Drawing for the job (mm, zero at the part's lowest x, y, z). Give positions to 0.01 mm unless a question says otherwise; leave off trailing zeros. Write each loop counter-clockwise with the first axis right and the second up, starting at its lowest first coordinate (ties: lowest second). Pieces come first, ordered by that corner, then holes.
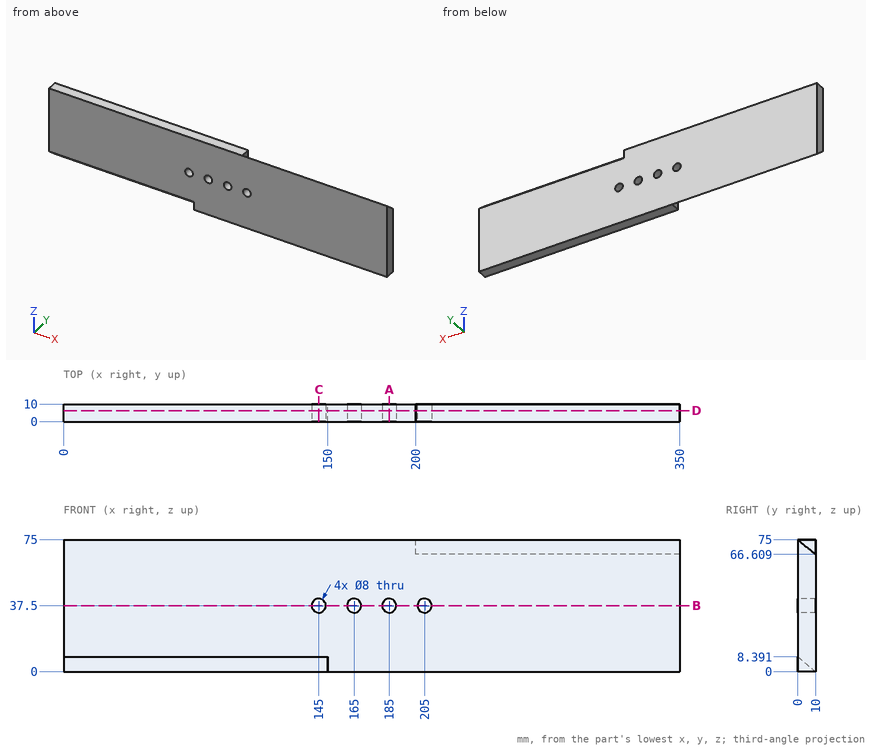
1. Slice it at C-C, the plane x = 145. Write the cut outline in (y, z).
Calculated:
outline: (0, 8.39) - (10, 0) - (10, 33.5) - (0, 33.5) - close; (0, 41.5) - (10, 41.5) - (10, 75) - (0, 75) - close
2. Slice it at D-D, the plane y = 6.25. Write the cut outline in (x, z), and give its area (3 significant figures).
Calculated:
outline: (0, 3.15) - (150, 3.15) - (150, 0) - (350, 0) - (350, 69.76) - (200, 69.76) - (200, 75) - (0, 75) - close; hole circle Ø8 at (145, 37.5); hole circle Ø8 at (165, 37.5); hole circle Ø8 at (185, 37.5); hole circle Ø8 at (205, 37.5)
area: 24,800 mm2
3. Pin check, flat tips, straight feed: P1, Ø8, axis at x = 113, z = 19.5, coming from the -Y side; P2, Ø6.5, axis at x = 145, z = 37.5, coming from the -Y side. Stop position of each tip, or through.
Calculated:
P1: stops at y = 0
P2: passes through
4. Slice it at B-B, the plane z = 37.5. Write the cut outline in (x, y).
Calculated:
outline: (0, 0) - (141, 0) - (141, 10) - (0, 10) - close; (149, 0) - (161, 0) - (161, 10) - (149, 10) - close; (169, 0) - (181, 0) - (181, 10) - (169, 10) - close; (189, 0) - (201, 0) - (201, 10) - (189, 10) - close; (209, 0) - (350, 0) - (350, 10) - (209, 10) - close
5. Slice it at A-A, the plane x = 185. Write the cut outline in (y, z), and give its area (3 significant figures).
Calculated:
outline: (0, 0) - (10, 0) - (10, 33.5) - (0, 33.5) - close; (0, 41.5) - (10, 41.5) - (10, 75) - (0, 75) - close
area: 670 mm2
6. Probe probe 1 along X at (y, z) = (4, 37.5); probe 2 along Z at (x, y) = (185, 2); probe 3 along X at (y, z) = (2, 39). List the from-to ranges inside material, lowest first.
Calculated:
probe 1: x = 0 to 141, 149 to 161, 169 to 181, 189 to 201, 209 to 350
probe 2: z = 0 to 33.5, 41.5 to 75
probe 3: x = 0 to 141.29, 148.71 to 161.29, 168.71 to 181.29, 188.71 to 201.29, 208.71 to 350
